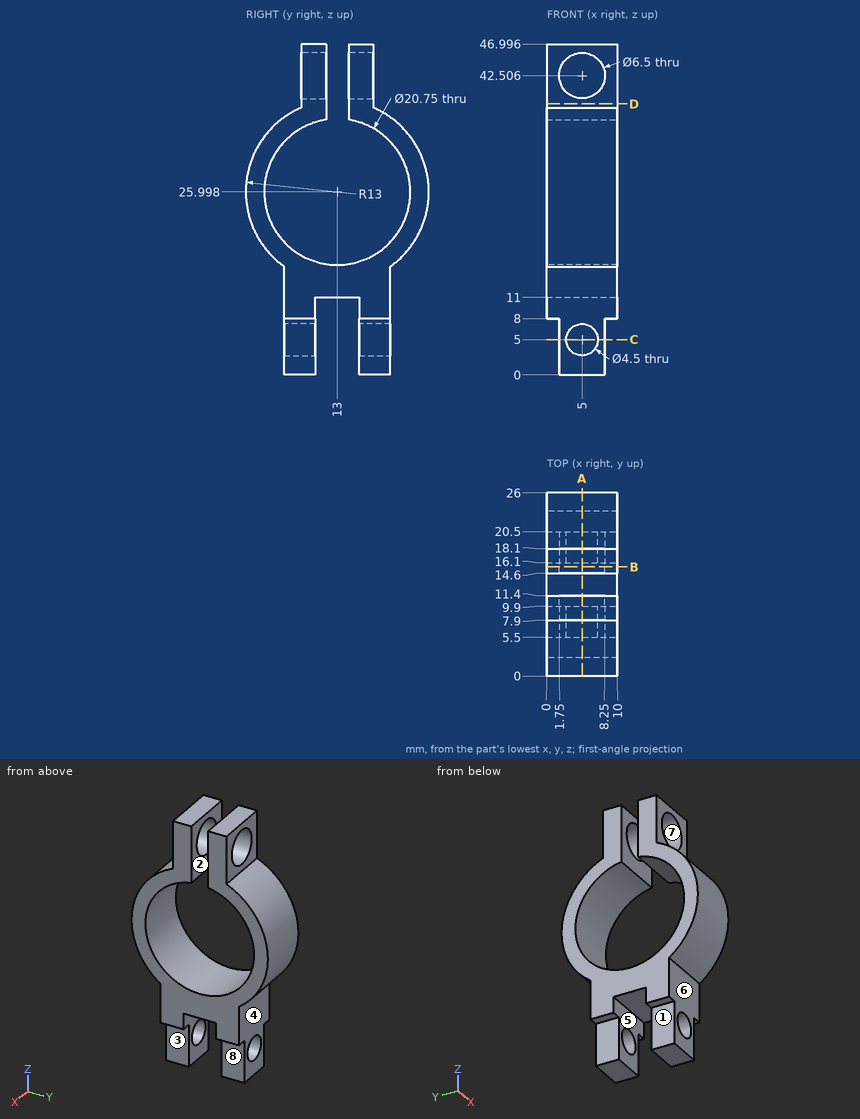
The figure shows three views and two pictorial views of one solid part (mm, origin at its lowest corner). Answer the questions. A direction names the side the tool comes from. Give positions to 0.01 mm unless a question says otherwise; leave off trailing zeros. Order: outer loops, then holes, each group sorted by start corner. A loop starts at its lowest first (then second) coordinate and runs counter-clockwise, first axis right, second up. Notation, with made-up numbers: M -6.5,20.25 L 1.5,20.25 A14 ccw 1.5,30.25 Z; hole C 77,19 d7. An arc over 180 degrees is marked long. Return JSON: item names as keys, results as strings.
1) Each of these flat-tipped pins is pushed along its axis until it touches: pin 1 (3 mm diameter, centred on x = 3.5, z = 5, fed in from +Y); pin 2 (1.9 mm diameter, centred on x = 9.5, y = 8, fed in from -Z); pin 3 (2 mm diameter, centred on y = 17.5, z = 4.5, fed in from +X). Where does it stop, or does it pass through?
Resolved:
{"pin 1": "y = 20.5", "pin 2": "z = 8", "pin 3": "x = 8.25"}
2) Straight lines are drawn through the part: line 1 along Y through (x, z) = (9, 40); line 2 along X through (y, z) = (19.3, 5); line 3 along Z through (x, y) = (2, 22) (1 decimal). For each, find the intervals that lie inside material, in ascending order. Write a range as [from, to].
Resolved:
{"line 1": "[7.9, 11.4], [14.6, 18.1]", "line 2": "[1.75, 2.75], [7.25, 8.25]", "line 3": "[16.6, 20.8], [31.2, 35.4]"}
3) Section B-B, the plane y = 15.5 is taken. Write down the section's boundary in (x, z), plus the area to 3 significant figures.
Resolved:
{"outline": "M 0,11 L 10,11 L 10,15.93 L 0,15.93 Z; M 0,36.07 L 10,36.07 L 10,47 L 0,47 Z; hole C 5,42.51 d6.5", "area": "125 mm^2"}
4) Section A-A, the plane x = 5 is taken. Give the number of separate pieces and of enclosed holes in the cut face, plus the area to 3 significant figures.
Resolved:
{"separate pieces": "5", "enclosed holes": "0", "area": "297 mm^2"}
5) A tool of negligible diameter and unlimited length cuts with its end or side. For the marked faces 1, 2, 3, 4 and 5, from which of +Z, -Z, +X, -X, +Y, -Y can it reach the whole face along a straight path? Write none if from no direction.
Resolved:
{"face 1": "-Z, -X, +Y, -Y", "face 2": "+Z, +X, -X", "face 3": "-Z, +X, +Y, -Y", "face 4": "-Z, +X, -X, +Y", "face 5": "-Z, +X, -X"}
6) For a pull along X with two mould halves and no side action, classify the marked faces 6, 7 and 8 as +X half, -X half, draft (parallel to the pull), parting line (faces both ways), or undercut.
Resolved:
{"face 6": "draft", "face 7": "undercut", "face 8": "+X half"}
7) Section D-D, the plane z = 38.5 is taken. Write down the section's boundary in (x, y).
Resolved:
{"outline": "M 0,7.9 L 10,7.9 L 10,11.4 L 0,11.4 Z; M 0,14.6 L 10,14.6 L 10,18.1 L 0,18.1 Z"}
8) Section C-C, the plane z = 5 is taken. Write down the section's boundary in (x, y), plus the area to 3 significant figures.
Resolved:
{"outline": "M 1.75,5.5 L 2.75,5.5 L 2.75,9.9 L 1.75,9.9 Z; M 1.75,16.1 L 2.75,16.1 L 2.75,20.5 L 1.75,20.5 Z; M 7.25,5.5 L 8.25,5.5 L 8.25,9.9 L 7.25,9.9 Z; M 7.25,16.1 L 8.25,16.1 L 8.25,20.5 L 7.25,20.5 Z", "area": "17.6 mm^2"}
